Autodesk Inventor part; units mm, degrees
ref_plane "YZ Plane" through (0, 0, 0) normal (1, 0, 0) x (0, 1, 0)
ref_plane "XZ Plane" through (0, 0, 0) normal (0, 1, 0) x (-1, 0, 0)
ref_plane "XY Plane" through (0, 0, 0) normal (0, 0, 1) x (1, 0, 0)
sketch "Sketch1" plane through (0, 0, 0) normal (0, 0, 1) x (1, 0, 0)
  circle A0 centre (0, 0) radius 65
  dimension "d0" = 130
extrude "Plate1" add sketch "Sketch1" against normal blind 3
sketch "Sketch2" plane through (0, 0, 0) normal (0, 0, 1) x (1, 0, 0)
  circle A0 centre (0, 55) radius 5
  circle A1 centre (0, 0) radius 65
  dimension "d2" = 10
  dimension "d3" = 55
extrude "Cut1" cut sketch "Sketch2" against normal through all contours A0
pattern_circular "Circular Pattern1" count 6 over 360 about axis through (0, 0, 0) along (0, 0, -1) of "Cut1"
sketch "Sketch3" plane through (0, 0, 0) normal (0, 0, 1) x (1, 0, 0)
  circle A0 centre (0, 0) radius 17.5
  dimension "d9" = 35
extrude "Extrusion1" cut sketch "Sketch3" against normal through all
equation "\"d4\" = Thickness"
equation "\"d1\" = Thickness"
equation "\"BendReliefWidth\" = Thickness"
equation "\"BendReliefDepth\" = 0.5 * Thickness"
equation "\"CornerReliefSize\" = 4 * Thickness"
equation "\"MinimumRemnant\" = 2 * Thickness"
equation "\"TransitionRadius\" = BendRadius"
equation "\"JacobiRadiusSize\" = BendRadius"
equation "\"GapSize\" = Thickness"
properties part number "TRM 041 flange" material "Stainless Steel"
Work out the finished part from the listing and answer in its coordinate system (mm). Round coordinates to 2 decimals unless told otherwise and drop trailing zeros. Write each loop counter-clockwise with the first axis right and the second up, starting at its lowest first coordinate (ties: lowest second). Pieces come first, ordered by that corner, then holes.
1) Consider probe 1 along Y at (x, z) = (0, -1.8); probe 2 along Y at (x, z) = (2, -0.85); probe 3 along X at (y, z) = (-0.5, -1.55). Determine where each line is inside the solid, lowest interval first.
2) A cutting plane is placed at B-B on y = 30. Determine the outline of the cut face in (x, z).
3) A cutting plane is placed at C-C on x = 48.5. Determine the outline of the cut face in (y, z).
4) Determine the mould class of faces 1 (the face through (-51.3, -24.1, -1.5)), 2 (the face through (46.55, -32.38, -1.48)), 3 (the face through (62, 19.52, -1.48)), 4 (the face through (14, -14, 0)) for opening direction X: pulls with the +X half, pulls with the -X half, needs draft (parallel to the pull), parting line crosses it, or undercut.
5) A cutting plane is placed at A-A on y = 0. Determine the outline of the cut face in (x, z), and give its area (3 significant figures).
6) Flat-ended cylindrical pins translate along their axes: P1, Ø9, axis at x = 0, y = -55, coming from the +Z side; P2, Ø1.5, axis at y = -28, z = -2.5, coming from the -X side. Find the tip coordinate at first contact, or state that the pin passes through.
7) A cutting plane is placed at D-D on z = -2.2. Determine the outline of the cut face in (x, y).
Entries:
1. probe 1: y = -65 to -60, -50 to -17.5, 17.5 to 50, 60 to 65
1. probe 2: y = -64.97 to -59.58, -50.42 to -17.39, 17.39 to 50.42, 59.58 to 64.97
1. probe 3: x = -65 to -17.49, 17.49 to 65
2. outline: (-57.66, -3) - (-51.96, -3) - (-51.96, 0) - (-57.66, 0) - close; (-43.3, -3) - (43.3, -3) - (43.3, 0) - (-43.3, 0) - close; (51.96, -3) - (57.66, -3) - (57.66, 0) - (51.96, 0) - close
3. outline: (-43.28, -3) - (-32.42, -3) - (-32.42, 0) - (-43.28, 0) - close; (-22.58, -3) - (22.58, -3) - (22.58, 0) - (-22.58, 0) - close; (32.42, -3) - (43.28, -3) - (43.28, 0) - (32.42, 0) - close
4. face 1: undercut
4. face 2: undercut
4. face 3: parting line crosses it
4. face 4: needs draft
5. outline: (-65, -3) - (-17.5, -3) - (-17.5, 0) - (-65, 0) - close; (17.5, -3) - (65, -3) - (65, 0) - (17.5, 0) - close
5. area: 285 mm2
6. P1: passes through
6. P2: stops at x = -59.01
7. outline: circle Ø130 at (0, 0); hole circle Ø10 at (-47.63, -27.5); hole circle Ø10 at (-47.63, 27.5); hole circle Ø35 at (0, 0); hole circle Ø10 at (0, -55); hole circle Ø10 at (0, 55); hole circle Ø10 at (47.63, -27.5); hole circle Ø10 at (47.63, 27.5)
